Source: three-view drawing plus pictorial views. Frame: mm from the lowest corner of the part. A direction names the side the tool comes from. Give positions to 0.01 mm unless a question says otherwise; leave off trailing zeros. Order: outer loops, then holes, each group sorted by start corner. A loop starts at its lowest first (then second) coordinate and runs counter-clockwise, first axis right, second up. Notation, with made-up numbers: (56, 75) -> (89, 75) arc R31 cw to (89, 104) -> close; hole circle Ø9 at (-36.75, 31.5). An arc over 180 degrees is marked (long way). Answer in a Markdown table with one row per item.
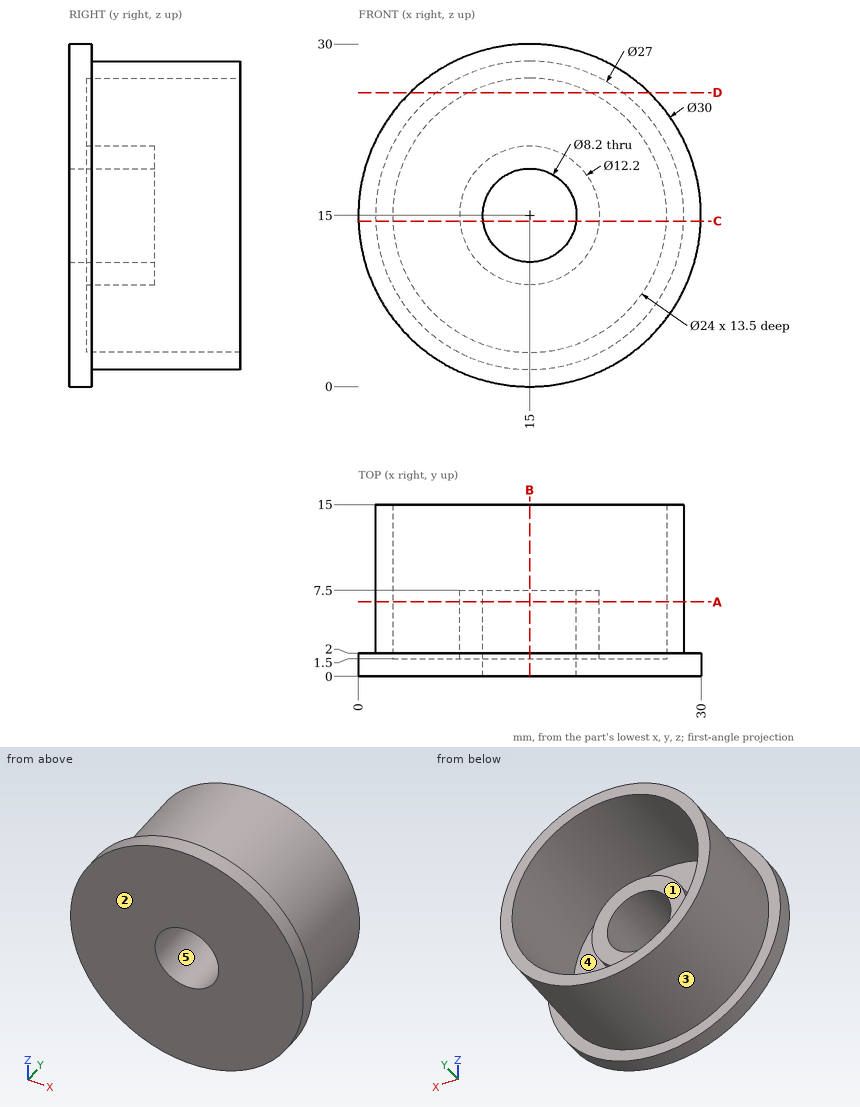
(1) Ray query, probe 1 along X at (y, z) = (5.25, 15); probe 2 along X at (y, z) = (8.25, 15); probe 3 along X at (y, z) = (4.5, 20.5). Return the intervals inside material, ascending.
A:
| item | result |
|---|---|
| probe 1 | x = 1.5 to 3, 8.9 to 10.9, 19.1 to 21.1, 27 to 28.5 |
| probe 2 | x = 1.5 to 3, 27 to 28.5 |
| probe 3 | x = 2.67 to 4.33, 12.36 to 17.64, 25.67 to 27.33 |
(2) Section query A-A (y = 6.5). Return the cut outline in (x, z).
A:
| item | result |
|---|---|
| outline | circle Ø27 at (15, 15); circle Ø12.2 at (15, 15); hole circle Ø24 at (15, 15); hole circle Ø8.2 at (15, 15) |
(3) Section query D-D (z = 25.75). Return the cut outline in (x, y).
A:
| item | result |
|---|---|
| outline | (4.54, 0) -> (25.46, 0) -> (25.46, 2) -> (23.17, 2) -> (23.17, 15) -> (20.33, 15) -> (20.33, 1.5) -> (9.67, 1.5) -> (9.67, 15) -> (6.83, 15) -> (6.83, 2) -> (4.54, 2) -> close |
(4) First-contact query: pin 1 Ø1.5 at (x, y) = (21.5, 6.5) entering from -Z; pin 2 Ø6 at (x, z) = (18, 18) entering from +Y; pin 3 Ø3 at (x, z) = (21.5, 21) entering from +Y. Flat tips, straight axial feed; report the tip coordinate or a pass-through.
A:
| item | result |
|---|---|
| pin 1 | stops at z = 2.79 |
| pin 2 | stops at y = 7.5 |
| pin 3 | stops at y = 1.5 |
(5) Access query for the marked faces 4 and 5. Directions: +Z, -Z, +X, -X, +Y, -Y. A direction counts if a zero-diameter tool reaches every point of the face in a straight line with its end or side. Return the directions, or none.
A:
| item | result |
|---|---|
| face 4 | +Y |
| face 5 | +Y, -Y |
(6) Section query C-C (z = 14.5). Return the cut outline in (x, y).
A:
| item | result |
|---|---|
| outline | (0.01, 0) -> (10.93, 0) -> (10.93, 7.5) -> (8.92, 7.5) -> (8.92, 1.5) -> (3.01, 1.5) -> (3.01, 15) -> (1.51, 15) -> (1.51, 2) -> (0.01, 2) -> close; (19.07, 0) -> (29.99, 0) -> (29.99, 2) -> (28.49, 2) -> (28.49, 15) -> (26.99, 15) -> (26.99, 1.5) -> (21.08, 1.5) -> (21.08, 7.5) -> (19.07, 7.5) -> close |
(7) Pull-direction query (X, two-part tool) for the marked faces 1, 2 and 3; classes: +X half, -X half, draft (parallel to the pull), parting line (faces both ways), or undercut.
A:
| item | result |
|---|---|
| face 1 | undercut |
| face 2 | draft |
| face 3 | parting line |
(8) Section query B-B (x = 15). Return the cut outline in (y, z).
A:
| item | result |
|---|---|
| outline | (0, 0) -> (2, 0) -> (2, 1.5) -> (15, 1.5) -> (15, 3) -> (1.5, 3) -> (1.5, 8.9) -> (7.5, 8.9) -> (7.5, 10.9) -> (0, 10.9) -> close; (0, 19.1) -> (7.5, 19.1) -> (7.5, 21.1) -> (1.5, 21.1) -> (1.5, 27) -> (15, 27) -> (15, 28.5) -> (2, 28.5) -> (2, 30) -> (0, 30) -> close |
